from build123d import *

# Parameters (mm, degrees)
SKETCH1_W           = 76
SKETCH1_H           = 10
BOSS_EXTRUDE1_DEPTH = 30
BOSS_EXTRUDE2_DEPTH = 18
CUT_EXTRUDE1_REACH  = 59.518
SKETCH12_4_R        = 8
CUT_EXTRUDE2_DEPTH  = 58.518373937
SKETCH12_5_R        = 8
CUT_EXTRUDE3_DEPTH  = 4
FILLET1_R           = 10


with BuildPart() as part:
    # Sketch1 → Boss-Extrude1 (new, symmetric)
    with BuildSketch(Plane.XY):
        Rectangle(SKETCH1_W, SKETCH1_H)
    extrude(amount=BOSS_EXTRUDE1_DEPTH, both=True)

    # Sketch1_4 → Boss-Extrude2 (add, symmetric)
    with BuildSketch(Plane.XY):
        Polygon((-16.502172006, 24.837168313), (-23.722310804, 5), (38, 5), align=None)
    extrude(amount=BOSS_EXTRUDE2_DEPTH, both=True)

    # Cut-Extrude1: up to this plane
    cut_extrude1_end = Plane(origin=(0, 5, 30), z_dir=(0, 1, 0))
    # Sketch2 → Cut-Extrude1 (cut, up to the surface)
    with BuildSketch(Plane(origin=(6.052124605, 16.628075692, 0), x_dir=(0.9396926207859105, -0.34202014332566305, 0), z_dir=(0.34202014332566305, 0.9396926207859105, 0)), mode=Mode.PRIVATE) as cut_extrude1_sk1:
        with BuildLine():
            Line((-6.001781127, 18), (-24.001781127, 18))
            Line((-24.001781127, 18), (-24.001781127, -2e-09))
            ThreePointArc((-24.001781127, -2e-09), (-23.938730537, 1.505272684), (-23.750020476, 3))
            ThreePointArc((-23.750020476, 3), (-18.729703188, 12.727922061), (-9.001781127, 17.748239349))
            ThreePointArc((-9.001781127, 17.748239349), (-7.507053812, 17.93694941), (-6.001781127, 18))
        make_face()
    cut_extrude1_tool1 = split(extrude(cut_extrude1_sk1.sketch, amount=-CUT_EXTRUDE1_REACH, mode=Mode.PRIVATE), bisect_by=cut_extrude1_end, keep=Keep.BOTH, mode=Mode.PRIVATE)
    add(cut_extrude1_tool1.solids().sort_by_distance((-12.724022, 23.462034, -13.979377))[0], mode=Mode.SUBTRACT)
    # Sketch2 → Cut-Extrude1 (cut, up to the surface)
    with BuildSketch(Plane(origin=(6.052124605, 16.628075692, 0), x_dir=(0.9396926207859105, -0.34202014332566305, 0), z_dir=(0.34202014332566305, 0.9396926207859105, 0)), mode=Mode.PRIVATE) as cut_extrude1_sk2:
        with BuildLine():
            ThreePointArc((-23.890324947, -2), (-23.973895481, -1.001551607), (-24.001781127, -2e-09))
            Line((-24.001781127, -2e-09), (-24.001781127, -18))
            Line((-24.001781127, -18), (-6.001781127, -18))
            ThreePointArc((-6.001781127, -18), (-7.507053812, -17.93694941), (-9.001781127, -17.748239349))
            ThreePointArc((-9.001781127, -17.748239349), (-19.081711416, -12.365897607), (-23.890324947, -2))
        make_face()
    cut_extrude1_tool2 = split(extrude(cut_extrude1_sk2.sketch, amount=-CUT_EXTRUDE1_REACH, mode=Mode.PRIVATE), bisect_by=cut_extrude1_end, keep=Keep.BOTH, mode=Mode.PRIVATE)
    add(cut_extrude1_tool2.solids().sort_by_distance((-12.724022, 23.462034, 13.979377))[0], mode=Mode.SUBTRACT)

    # Sketch12_4 → Cut-Extrude2 (cut, through all)
    with BuildSketch(Plane(origin=(6.052124605, 16.628075692, 0), x_dir=(0.9396926207859105, -0.34202014332566305, 0), z_dir=(0.34202014332566305, 0.9396926207859105, 0))):
        with Locations(Location((-6.001781127, 0, 0), (0, 0, 180))):
            Circle(SKETCH12_4_R)
    extrude(amount=-CUT_EXTRUDE2_DEPTH, mode=Mode.SUBTRACT)

    # Sketch12_5 → Cut-Extrude3 (cut)
    with BuildSketch(Plane(origin=(6.052124605, 16.628075692, 0), x_dir=(0.9396926207859105, -0.34202014332566305, 0), z_dir=(0.34202014332566305, 0.9396926207859105, 0))):
        with BuildLine():
            ThreePointArc((-23.750020476, 3), (-23.938730537, 1.505272688), (-24.001781127, 5e-09))
            ThreePointArc((-24.001781127, 5e-09), (-23.973895482, -1.001551604), (-23.890324947, -2))
            Line((-23.890324947, -2), (-18.847013705, -2))
            ThreePointArc((-18.847013705, -2), (-15.547394686, -8.825036078), (-9.001781127, -12.649110641))
            Line((-9.001781127, -12.649110641), (-9.001781127, -17.748239349))
            ThreePointArc((-9.001781127, -17.748239349), (-7.507053812, -17.93694941), (-6.001781127, -18))
            Line((-6.001781127, -18), (-4.001781127, -18))
            Line((-4.001781127, -18), (-4.001781127, -12.845232579))
            ThreePointArc((-4.001781127, -12.845232579), (3.190607029, -9.192388155), (6.843451452, -2))
            Line((6.843451452, -2), (33.998218873, -2))
            Line((33.998218873, -2), (33.998218873, 3))
            Line((33.998218873, 3), (6.647329514, 3))
            ThreePointArc((6.647329514, 3), (2.823254951, 9.54561356), (-4.001781127, 12.845232579))
            Line((-4.001781127, 12.845232579), (-4.001781127, 18))
            Line((-4.001781127, 18), (-6.001781127, 18))
            ThreePointArc((-6.001781127, 18), (-7.507053812, 17.93694941), (-9.001781127, 17.748239349))
            Line((-9.001781127, 17.748239349), (-9.001781127, 12.649110641))
            ThreePointArc((-9.001781127, 12.649110641), (-15.194169282, 9.192388155), (-18.650891767, 3))
            Line((-18.650891767, 3), (-23.750020476, 3))
        make_face()
        with Locations(Location((-6.001781127, 0, 0), (0, 0, 180))):
            Circle(SKETCH12_5_R, mode=Mode.SUBTRACT)
    extrude(amount=-CUT_EXTRUDE3_DEPTH, mode=Mode.SUBTRACT)

    # Fillet1
    fillet1_edges = [part.edges().sort_by_distance(p)[0] for p in [
        (38, 0, 30),
        (-38, 0, 30),
        (38, 0, -30),
        (-38, 0, -30),
    ]]
    fillet(fillet1_edges, radius=FILLET1_R)


solid = part.part
Read the model definition and answer for the solid it produces. Units are mm, in the model's axes. A direction names the side the tool comes from. Round coordinates to 2 decimals unless told otherwise and drop trailing zeros. Write each loop counter-clockwise with the first axis right and the second up, starting at its lowest first coordinate (ties: lowest second). Pieces come first, ordered by that corner, then holes.
Q1. Find section A-A on z = -2. Determine the outline of the cut face in (x, y).
Values:
outline: (-38, -5) - (-16.45, -5) - (-8.23, 17.57) - (-17.77, 21.04) - (-23.6, 5) - (-38, 5) - close; (0.04, -5) - (38, -5) - (38, 5) - (36.63, 1.24) - (6.32, 12.27) - close
Q2. The mould has two halves that part along Z. Classify faces 1 (the face through (0, 0, 30)), 2 (the face through (-8.833, 19.947, -9.263)), 3 (the face through (24.363, 9.963, 10.112)): released by +Z, released by -Z, zero draft, split by the parting line, or undercut.
Values:
face 1: released by +Z
face 2: undercut
face 3: zero draft
Q3. A tool of negligible diameter and unlimited length cuts with its end or side. For faces 4 (the face through (-3.081, 17.854, 15.163)), 5 (the face through (-15, 22, 2)), 6 (the face through (25, 8, -3)), from which of +Z, -Z, +X, -X, +Y, -Y can it reach the whole face along a straight path? Write none if from no direction.
Values:
face 4: +Z, -Z
face 5: +X, +Y
face 6: +Y
Q4. Flat-ended cylindrical pins translate along their axes: P1, Ø2.5, axis at x = -15.5, y = 22.5, coming from the -Z side; P2, Ø4, axis at y = 21, z = 1.5, coming from the +X side; P3, Ø3, axis at x = -4.5, y = 11, coming from the +Z side. Find the tip coordinate at first contact, or state that the pin passes through.
Values:
P1: stops at z = -9.94
P2: stops at x = -11.69
P3: stops at z = 17.99
Q5. Find section D-D on y = 3.5. State how many separate pieces and enclosed holes the cut face has, and give its area (3 significant figures).
Values:
separate pieces: 1
enclosed holes: 2
area: 4,230 mm2
Q6. Find section C-C on z = -16. Determine the outline of the cut face in (x, y).
Values:
outline: (-38, -5) - (38, -5) - (38, 5) - (2.29, 18) - (0.92, 14.24) - (-3.77, 15.95) - (-2.41, 19.71) - (-7.34, 21.5) - (-13.34, 5) - (-38, 5) - close
Q7. Straight lines are drawn through the part: line 1 (Y direction, x = -15, z = 27.5); line 2 (Z direction, x = -3, y = 7.25); line 3 (Z direction, x = 2.5, y = 12.75). For each, find the intervals that lie inside material, in ascending order.
Values:
line 1: y = -5 to 5
line 2: z = -18 to -7.97, 7.97 to 18
line 3: z = -18 to -6.93, 6.93 to 18
Q8. Find section B-B on x = 32.5. Determine the outline of the cut face in (y, z), and give its area (3 significant figures).
Values:
outline: (-5, -28.93) - (5, -28.93) - (5, -18) - (7, -18) - (7, -3) - (2.75, -3) - (2.75, 2) - (7, 2) - (7, 18) - (5, 18) - (5, 28.93) - (-5, 28.93) - close
area: 629 mm2
